Design review of the part built by this model. Coordinates are the model's own, in mm. Face numbers are marked on the shaded views. A direction names the side the tool comes from. Give positions to 0.01 mm unless a question says otherwise; leave off trailing zeros. Loops run counter-clockwise (first coordinate to the right, second up) from the corner with the lowest first, then second, coordinate; pieces in that order, holes last. Notation, with made-up numbers: (71, 71) - (130, 71) arc R37 cw to (130, 109) - close; hole circle Ø7 at (24.5, -20). An arc over 180 degrees is marked (long way). One line per item, written item: value. Start each with the question number.
```python
from build123d import *

# Parameters (mm, degrees)
F1_DEPTH = 10
F2_R     = 1.5
F3_DEPTH = 10.001


with BuildPart() as f1:
    # F0 (on Top) → F1 (new body)
    with BuildSketch(Plane.XY):
        with BuildLine():
            ThreePointArc((10.305245, -2.586998), (10.544758, -1.303342), (10.625, 0))
            ThreePointArc((10.625, 0), (10.623229, 0.193975), (10.617917, 0.387885))
            ThreePointArc((10.617917, 0.387885), (10.566795, 1.110615), (10.466536, 1.82818))
            ThreePointArc((10.466536, 1.82818), (10.104975, 3.283306), (9.542183, 4.673047))
            ThreePointArc((9.542183, 4.673047), (9.20152, 5.3125), (8.818069, 5.927249))
            ThreePointArc((8.818069, 5.927249), (7.895914, 7.109513), (6.816518, 8.150196))
            ThreePointArc((6.816518, 8.150196), (6.245218, 8.595806), (5.644877, 9.001444))
            ThreePointArc((5.644877, 9.001444), (4.321577, 9.70642), (2.912216, 10.218103))
            ThreePointArc((2.912216, 10.218103), (2.209062, 10.392818), (1.495635, 10.519206))
            ThreePointArc((1.495635, 10.519206), (0, 10.625), (-1.495635, 10.519206))
            ThreePointArc((-1.495635, 10.519206), (-2.209062, 10.392818), (-2.912216, 10.218103))
            ThreePointArc((-2.912216, 10.218103), (-4.321577, 9.70642), (-5.644877, 9.001444))
            ThreePointArc((-5.644877, 9.001444), (-6.245218, 8.595806), (-6.816518, 8.150196))
            ThreePointArc((-6.816518, 8.150196), (-7.895914, 7.109513), (-8.818069, 5.927249))
            ThreePointArc((-8.818069, 5.927249), (-9.20152, 5.3125), (-9.542183, 4.673047))
            ThreePointArc((-9.542183, 4.673047), (-10.104975, 3.283306), (-10.466536, 1.82818))
            ThreePointArc((-10.466536, 1.82818), (-10.566795, 1.110615), (-10.617917, 0.387885))
            ThreePointArc((-10.617917, 0.387885), (-10.566795, -1.110615), (-10.305245, -2.586998))
            ThreePointArc((-10.305245, -2.586998), (-10.104975, -3.283306), (-9.857717, -3.964345))
            ThreePointArc((-9.857717, -3.964345), (-9.20152, -5.3125), (-8.362082, -6.554861))
            ThreePointArc((-8.362082, -6.554861), (-7.895914, -7.109513), (-7.393029, -7.631104))
            ThreePointArc((-7.393029, -7.631104), (-6.245218, -8.595806), (-4.97304, -9.389329))
            ThreePointArc((-4.97304, -9.389329), (-4.321577, -9.70642), (-3.650018, -9.978376))
            ThreePointArc((-3.650018, -9.978376), (-2.209062, -10.392818), (-0.724114, -10.600296))
            ThreePointArc((-0.724114, -10.600296), (0, -10.625), (0.724114, -10.600296))
            ThreePointArc((0.724114, -10.600296), (2.209062, -10.392818), (3.650018, -9.978376))
            ThreePointArc((3.650018, -9.978376), (4.321577, -9.70642), (4.97304, -9.389329))
            ThreePointArc((4.97304, -9.389329), (6.245218, -8.595806), (7.393029, -7.631104))
            ThreePointArc((7.393029, -7.631104), (7.895914, -7.109513), (8.362082, -6.554861))
            ThreePointArc((8.362082, -6.554861), (9.20152, -5.3125), (9.857717, -3.964345))
            ThreePointArc((9.857717, -3.964345), (10.104975, -3.283306), (10.305245, -2.586998))
        make_face()
        with BuildLine():
            ThreePointArc((10.617917, 0.387885), (10.623229, 0.193975), (10.625, 0))
            ThreePointArc((10.625, 0), (10.544758, -1.303342), (10.305245, -2.586998))
            Line((10.305245, -2.586998), (13.471964, -2.170092))
            Line((13.471964, -2.170092), (13.550361, -1.4242))
            Line((13.550361, -1.4242), (13.628757, -0.678309))
            Line((13.628757, -0.678309), (10.617917, 0.387885))
        make_face()
        with BuildLine():
            ThreePointArc((9.542183, 4.673047), (10.104975, 3.283306), (10.466536, 1.82818))
            Line((10.466536, 1.82818), (13.189908, 3.497064))
            Line((13.189908, 3.497064), (12.958145, 4.210357))
            Line((12.958145, 4.210357), (12.726382, 4.923649))
            Line((12.726382, 4.923649), (9.542183, 4.673047))
        make_face()
        with BuildLine():
            Line((12.174596, -6.162981), (9.857717, -3.964345))
            ThreePointArc((9.857717, -3.964345), (9.20152, -5.3125), (8.362082, -6.554861))
            Line((8.362082, -6.554861), (11.424596, -7.462019))
            Line((11.424596, -7.462019), (11.799596, -6.8125))
            Line((11.799596, -6.8125), (12.174596, -6.162981))
        make_face()
        with BuildLine():
            ThreePointArc((6.816518, 8.150196), (7.895914, 7.109513), (8.818069, 5.927249))
            Line((8.818069, 5.927249), (10.627196, 8.559546))
            Line((10.627196, 8.559546), (10.125348, 9.116905))
            Line((10.125348, 9.116905), (9.6235, 9.674263))
            Line((9.6235, 9.674263), (6.816518, 8.150196))
        make_face()
        with BuildLine():
            Line((8.615337, -10.582018), (7.393029, -7.631104))
            ThreePointArc((7.393029, -7.631104), (6.245218, -8.595806), (4.97304, -9.389329))
            Line((4.97304, -9.389329), (7.401811, -11.463695))
            Line((7.401811, -11.463695), (8.008574, -11.022857))
            Line((8.008574, -11.022857), (8.615337, -10.582018))
        make_face()
        with BuildLine():
            ThreePointArc((2.912216, 10.218103), (4.321577, 9.70642), (5.644877, 9.001444))
            Line((5.644877, 9.001444), (6.226946, 12.142004))
            Line((6.226946, 12.142004), (5.541787, 12.447057))
            Line((5.541787, 12.447057), (4.856628, 12.752109))
            Line((4.856628, 12.752109), (2.912216, 10.218103))
        make_face()
        with BuildLine():
            Line((3.566407, -13.171327), (3.650018, -9.978376))
            ThreePointArc((3.650018, -9.978376), (2.209062, -10.392818), (0.724114, -10.600296))
            Line((0.724114, -10.600296), (2.099186, -13.483195))
            Line((2.099186, -13.483195), (2.832797, -13.327261))
            Line((2.832797, -13.327261), (3.566407, -13.171327))
        make_face()
        with BuildLine():
            ThreePointArc((-1.495635, 10.519206), (0, 10.625), (1.495635, 10.519206))
            Line((1.495635, 10.519206), (0.75, 13.625))
            Line((0.75, 13.625), (0, 13.625))
            Line((0, 13.625), (-0.75, 13.625))
            Line((-0.75, 13.625), (-1.495635, 10.519206))
        make_face()
        with BuildLine():
            Line((-2.099186, -13.483195), (-0.724114, -10.600296))
            ThreePointArc((-0.724114, -10.600296), (-2.209062, -10.392818), (-3.650018, -9.978376))
            Line((-3.650018, -9.978376), (-3.566407, -13.171327))
            Line((-3.566407, -13.171327), (-2.832797, -13.327261))
            Line((-2.832797, -13.327261), (-2.099186, -13.483195))
        make_face()
        with BuildLine():
            ThreePointArc((-5.644877, 9.001444), (-4.321577, 9.70642), (-2.912216, 10.218103))
            Line((-2.912216, 10.218103), (-4.856628, 12.752109))
            Line((-4.856628, 12.752109), (-5.541787, 12.447057))
            Line((-5.541787, 12.447057), (-6.226946, 12.142004))
            Line((-6.226946, 12.142004), (-5.644877, 9.001444))
        make_face()
        with BuildLine():
            Line((-7.401811, -11.463695), (-4.97304, -9.389329))
            ThreePointArc((-4.97304, -9.389329), (-6.245218, -8.595806), (-7.393029, -7.631104))
            Line((-7.393029, -7.631104), (-8.615337, -10.582018))
            Line((-8.615337, -10.582018), (-8.008574, -11.022857))
            Line((-8.008574, -11.022857), (-7.401811, -11.463695))
        make_face()
        with BuildLine():
            ThreePointArc((-8.818069, 5.927249), (-7.895914, 7.109513), (-6.816518, 8.150196))
            Line((-6.816518, 8.150196), (-9.6235, 9.674263))
            Line((-9.6235, 9.674263), (-10.125348, 9.116905))
            Line((-10.125348, 9.116905), (-10.627196, 8.559546))
            Line((-10.627196, 8.559546), (-8.818069, 5.927249))
        make_face()
        with BuildLine():
            Line((-11.424596, -7.462019), (-8.362082, -6.554861))
            ThreePointArc((-8.362082, -6.554861), (-9.20152, -5.3125), (-9.857717, -3.964345))
            Line((-9.857717, -3.964345), (-12.174596, -6.162981))
            Line((-12.174596, -6.162981), (-11.799596, -6.8125))
            Line((-11.799596, -6.8125), (-11.424596, -7.462019))
        make_face()
        with BuildLine():
            ThreePointArc((-10.466536, 1.82818), (-10.104975, 3.283306), (-9.542183, 4.673047))
            Line((-9.542183, 4.673047), (-12.726382, 4.923649))
            Line((-12.726382, 4.923649), (-12.958145, 4.210357))
            Line((-12.958145, 4.210357), (-13.189908, 3.497064))
            Line((-13.189908, 3.497064), (-10.466536, 1.82818))
        make_face()
        with BuildLine():
            Line((-13.471964, -2.170092), (-10.305245, -2.586998))
            ThreePointArc((-10.305245, -2.586998), (-10.566795, -1.110615), (-10.617917, 0.387885))
            Line((-10.617917, 0.387885), (-13.628757, -0.678309))
            Line((-13.628757, -0.678309), (-13.550361, -1.4242))
            Line((-13.550361, -1.4242), (-13.471964, -2.170092))
        make_face()
    extrude(amount=F1_DEPTH)

    # F2 (on face) → F3 (cut, through all)
    with BuildSketch(Plane.XY.offset(10)):
        Circle(F2_R)
    extrude(amount=-F3_DEPTH, mode=Mode.SUBTRACT)


solid = f1.part
```
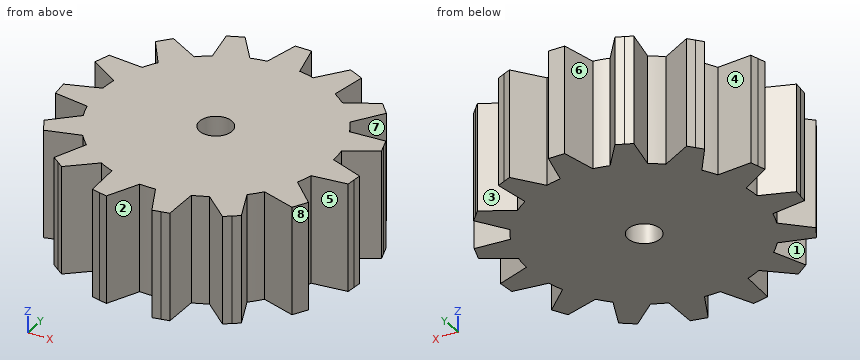
(1) Take a section at C-C on y = -9. State the section outline as (x, z) points.
(2) For pin 1 Ø5 at (y, z) = (-6, 4.5) entering from +X; pin 2 Ø5 at (x, y) = (-1, 0.5) entering from -Z; pin 3 Ø1.5 at (x, z) = (2.5, 4) entering from +Y, all flat-tipped, find the tip position at first contact; note any pin that passes through.
(3) Take a section at A-A on x = 0. State the section outline as (y, z) points (3 decimals), and give its area (4 significant figures).
(4) Machinability: for the marked faces 1, 2, 3, 4 and 5, which of the approach directions +Z, -Z, +X, -X, +Y, -Y give a long, thin tool a straight path to every point of the face, cutting with its end or side? Answer none if there is none.
(5) Draft analysis for pull direction Y (two halves, no side actions). For the marked faces 6, 7 and 8, state which applies: pulls with the +Y half, pulls with the -Y half, needs draft (parallel to the pull), parting line crosses it, or undercut.
(6) To check wall thickness, follow L1, parallel to Y at x = 0, z = 6.25 (3 decimals); L2, parallel to X at y = 11.5, z = 4.5; L3, parallel to X at y = 8.5, z = 1 (3 decimals). State the ranges of each line that lie inside material, in increasing order. Write a range as from..to.
(7) Take a section at B-B on y = 0. State the section outline as (x, z) points, and give its area (3 significant figures).
Here are the results:
1. outline: (-7.96, 0) - (7.96, 0) - (7.96, 10) - (-7.96, 10) - close
2. pin 1: x = 12.17
2. pin 2: z = 0
2. pin 3: y = 10.66
3. outline: (-10.625, 0) - (-1.5, 0) - (-1.5, 10) - (-10.625, 10) - close; (1.5, 0) - (13.625, 0) - (13.625, 10) - (1.5, 10) - close
3. area: 212.5 mm²
4. face 1: +Z, -Z, -X
4. face 2: +Z, -Z, -Y
4. face 3: +Z, -Z, +Y
4. face 4: +Z, -Z
4. face 5: +Z, -Z, +X
5. face 6: pulls with the +Y half
5. face 7: undercut
5. face 8: pulls with the -Y half
6. L1: -10.625..-1.5, 1.5..13.625
6. L2: -6.11..-3.9, -1.26..1.26, 3.9..6.11
6. L3: -10.586..-7.461, -6.375..6.375, 7.461..10.586
7. outline: (-11.71, 0) - (-1.5, 0) - (-1.5, 10) - (-11.71, 10) - close; (1.5, 0) - (11.71, 0) - (11.71, 10) - (1.5, 10) - close
7. area: 204 mm²
